```python
from build123d import *

# Parameters (mm, degrees)
F0_W     = 19.05
F0_H     = 19.05
F0_H_2   = 190.5
F0_H_3   = 279.4
F1_DEPTH = 431.8


with BuildPart() as f1:
    # F0 (on Front) → F1 (new body)
    with BuildSketch(Plane.XZ):
        with Locations((-393.7, 400.9142230511)):
            Rectangle(F0_W, F0_H)
        with Locations((-393.7, 296.1392230511)):
            Rectangle(F0_W, F0_H_2)
        with Locations((393.7, 400.9142230511)):
            Rectangle(F0_W, F0_H)
        with Locations((-393.7, 191.3642230511)):
            Rectangle(F0_W, F0_H)
        with Locations((393.7, 296.1392230511)):
            Rectangle(F0_W, F0_H_2)
        Polygon((-162.0973050594, 200.8892230511), (-384.175, 200.8892230511), (-384.175, 181.8392230511), (-162.0973050594, 181.8392230511), (384.175, 181.8392230511), (384.175, 200.8892230511), align=None)
        with Locations((-393.7, 42.1392230511)):
            Rectangle(F0_W, F0_H_3)
        with Locations((393.7, 191.3642230511)):
            Rectangle(F0_W, F0_H)
        with Locations((-393.7, -107.0857769489)):
            Rectangle(F0_W, F0_H)
        with Locations((393.7, 42.1392230511)):
            Rectangle(F0_W, F0_H_3)
        Polygon((-162.0973050594, -97.5607769489), (-384.175, -97.5607769489), (-384.175, -116.6107769489), (-162.0973050594, -116.6107769489), (384.175, -116.6107769489), (384.175, -97.5607769489), align=None)
        with Locations((-393.7, -256.3107769489)):
            Rectangle(F0_W, F0_H_3)
        with Locations((393.7, -107.0857769489)):
            Rectangle(F0_W, F0_H)
        with Locations((393.7, -256.3107769489)):
            Rectangle(F0_W, F0_H_3)
    extrude(amount=-F1_DEPTH)


solid = f1.part
```
Check sheet for the modelled part. Datum: model origin and axes. Units: mm. A direction names the side the tool comes from. Coordinates: 2 decimals unless noted, no trailing zeros. Write each loop counter-clockwise with the first axis right and the second up, starting at its lowest first coordinate (ties: lowest second). Pieces come first, ordered by that corner, then holes. Notation, with made-up numbers: M 43.5,66.25 L 59.5,66.25 A5 ccw 59.5,74.25 Z; hole C -22.5,-7.5 d3. An arc over 180 degrees is marked long. Write item = value, one per line. Start each with the question number.
1. Thickness scan on probe 1 along Z at (x, y) = (289, 218); probe 2 along X at (y, z) = (343, 35) (3 decimals). Record the ranges inside material, lowest first.
2. Mould release check, pull along X, two halves, no side actions. Record for faces 1 (the flat face through (394, 213, 410.439)), 2 (the flat face through (-403.225, 213, 13)), 3 (the flat face through (-384.175, 213, 304)): pulls with the +X half, pulls with the -X half, needs draft (parallel to the pull), parting line crosses it, or undercut.
3. Go/stop test with flat-tipped pins: pin 1 (1.5 mm diameter, centred on x = 166, y = 287.5, fed in from +Z); pin 2 (1 mm diameter, centred on x = 277.5, y = 255.5, fed in from -Z). Record where each tip stops, or that it passes through.
4. Sectioned sample at B-B (x = 192.5). Record the cut outline in (y, z), then the cut area to 3 significant figures.
5. Sectioned sample at A-A (z = -37). Record the cut outline in (x, y) (3 decimals), then the cut area to 3 significant figures.
6. Tool access check on faces 4 (the flat face through (384.175, 213, 40)), 5 (the flat face through (384.175, 213, 307)), 6 (the flat face through (-384.175, 213, -258)). Record the directions out of +Z, -Z, +X, -X, +Y, -Y that give a thin tool (end or side, any length) a straight path to the whole face; none if there is none.
7. Sectioned sample at C-C (y = 157). Record the cut outline in (x, z) (3 decimals), then the cut area to 3 significant figures.
The answers:
q1.probe_1 = -116.61 to -97.56, 181.84 to 200.89
q1.probe_2 = -403.225 to -384.175, 384.175 to 403.225
q2.face_1 = needs draft
q2.face_2 = pulls with the -X half
q2.face_3 = undercut
q3.pin_1 = 200.89
q3.pin_2 = -116.61
q4.outline = M 0,-116.61 L 431.8,-116.61 L 431.8,-97.56 L 0,-97.56 Z; M 0,181.84 L 431.8,181.84 L 431.8,200.89 L 0,200.89 Z
q4.area = 16,500 mm²
q5.outline = M -403.225,0 L -384.175,0 L -384.175,431.8 L -403.225,431.8 Z; M 384.175,0 L 403.225,0 L 403.225,431.8 L 384.175,431.8 Z
q5.area = 16,500 mm²
q6.face_4 = +Y, -Y
q6.face_5 = +Z, +Y, -Y
q6.face_6 = -Z, +Y, -Y
q7.outline = M -403.225,-396.011 L -384.175,-396.011 L -384.175,-116.611 L 384.175,-116.611 L 384.175,-396.011 L 403.225,-396.011 L 403.225,410.439 L 384.175,410.439 L 384.175,200.889 L -384.175,200.889 L -384.175,410.439 L -403.225,410.439 Z; hole M -384.175,-97.561 L 384.175,-97.561 L 384.175,181.839 L -384.175,181.839 Z
q7.area = 60,000 mm²
